from build123d import *

# Parameters (mm, degrees)
F0_W        = 59
F0_H        = 41
F1_DEPTH    = 22
F2_R        = 15
F3_DEPTH    = 76.2
F4_T        = 0.5
F4_T4_ANGLE = 180.000000001
F4_T6_ANGLE = 180.000000001


# Not quite as in the source:
# - a shell that OpenCascade refuses in one call is made with other operations: the cavity is built on its own and cut out


with BuildPart() as f1:
    # F0 (on Front) → F1 (new body)
    with BuildSketch(Plane.XZ):
        Rectangle(F0_W, F0_H)
    extrude(amount=-F1_DEPTH)

    # F2 (on Front) → F3 (join)
    with BuildSketch(Plane.XZ):
        with Locations((-14.5, 0)):
            Circle(F2_R)
    extrude(amount=-F3_DEPTH)

    # F4: shell of thickness 0.5, made by hand


with BuildPart() as f4_core1:
    # F4_t2: copy of F1
    add(f1.part)

    # the walls: a layer under each face that stays
    f4_faces = [f4_core1.faces().sort_by_distance(p)[0] for p in [
        (29.5, 11, 0),
        (0, 22, -13.6666666667),
        (-29.5, 49.1, 0),
        (-14.5, 76.2, 0),
        (-29.5, 11, 0),
        (0, 11, 20.5),
        (0, 11, -20.5),
    ]]
    thicken(f4_faces, amount=-F4_T, mode=Mode.SUBTRACT)

    # F4_s3 → F4_t4 (revolve, cut)
    with BuildSketch(Plane.XY):
        Polygon((-29.505, 22.005), (-29.5, 21.5), (-29, 21.5), (-29, 22), align=None)
    revolve(axis=Axis((-14.5, 22, 0), (0, -1, 0)), revolution_arc=F4_T4_ANGLE, mode=Mode.SUBTRACT)

    # F4_s5 → F4_t6 (revolve, cut)
    with BuildSketch(Plane.XY):
        Polygon((0.505, 22.005), (0.5, 21.5), (0, 21.5), (0, 22), align=None)
    revolve(axis=Axis((-14.5, 22, 0), (0, -1, 0)), revolution_arc=F4_T6_ANGLE, mode=Mode.SUBTRACT)


with BuildPart() as f1_1:
    add(f1.part)

    # what is left inside the walls is the cavity
    f4_cavity = [f4_core1.part.solids().sort_by_distance(p)[0] for p in [
        (-28.995, 57.8, 0),
    ]]
    add(f4_cavity, mode=Mode.SUBTRACT)


solid = f1_1.part
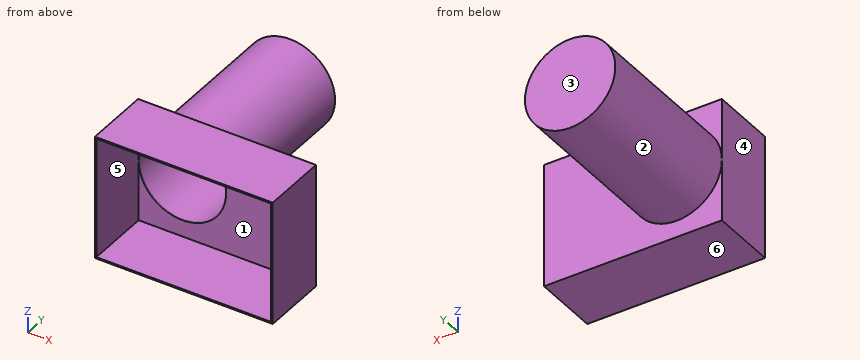
Geometry: final body of the model. Coordinates: model frame, mm. Face numbers are marked on the shaded views. A direction names the side the tool comes from. Give positions to 0.01 mm unless a question says otherwise; leave off trailing zeros. Loops run counter-clockwise (first coordinate to the right, second up) from the corner with the lowest first, then second, coordinate; pieces in that order, holes last. Notation, with made-up numbers: (17, -10.5) - (73, -10.5) arc R17 ccw to (73, 18.5) - close; hole circle Ø10 at (49.5, 28.25). An arc over 180 degrees is marked (long way). Answer as CSV lines item,"result". Start each with the question number.
1. Section D-D, the plane x = 10.5. Return loops of the section in (y, z), plus the area to 3 significant figures.
2. Reachability of the marked faces 1, 2 and 3 from +Z, -Z, +X, -X, +Y, -Y: full face, straight path, thin tool, end or side. Return the list, or none.
3. Section C-C, the plane z = -4.5. Return loops of the section in (x, y).
4. Draft query along Z for the marked faces 4, 5 and 6. Return one class per face: released by +Z, released by -Z, zero draft, split by the parting line, or undercut.
5. Section A-A, the plane y = 9. Return loops of the section in (x, z).
6. Section B-B, the plane x = -14.5. Return loops of the section in (y, z), plus the area to 3 significant figures.
7. Ray query, L1, parallel to X at y = 58, z = 0; L2, parallel to Z at x = -14.5, y = 56; L3, parallel to X at y = 6.5, z = 11.5. Return the intervals inside material, ascending.
8. Pin query (flat end, axial travel): P1, Ø6, axis at y = 48, z = -11, coming from the +X side; P2, Ø4, axis at x = 11.5, z = -3, coming from the -Y side; P3, Ø2, axis at x = -5, y = 39.5, coming from the -Z side. Return the tip coordinate at first contact, or that it passes through.
Answers:
1,outline,"(0, -20.5) - (22, -20.5) - (22, 20.5) - (0, 20.5) - (0, 20) - (21.5, 20) - (21.5, -20) - (0, -20) - close"
1,area,"42.0 mm2"
2,face 1,"-Y"
2,face 2,"+Y"
2,face 3,"+Z, -Z, +X, -X, +Y"
3,outline,"(-29.5, 0) - (-29, 0) - (-29, 21.5) - (-28.28, 21.5) - (-28.28, 75.7) - (-0.72, 75.7) - (-0.72, 21.5) - (29, 21.5) - (29, 0) - (29.5, 0) - (29.5, 22) - (-0.19, 22) - (-0.19, 76.2) - (-28.81, 76.2) - (-28.81, 22) - (-29.5, 22) - close"
4,face 4,"zero draft"
4,face 5,"undercut"
4,face 6,"released by -Z"
5,outline,"(-29.5, -20.5) - (29.5, -20.5) - (29.5, 20.5) - (-29.5, 20.5) - close; hole (-29, -20) - (29, -20) - (29, 20) - (-29, 20) - close"
6,outline,"(0, -20.5) - (22, -20.5) - (22, -15) - (76.2, -15) - (76.2, 15) - (22, 15) - (22, 20.5) - (0, 20.5) - (0, 20) - (21.5, 20) - (21.5, 14.5) - (75.7, 14.5) - (75.7, -14.5) - (21.5, -14.5) - (21.5, -20) - (0, -20) - close"
6,area,"96.2 mm2"
7,L1,"x = -29.5 to -29, 0 to 0.5"
7,L2,"z = -15 to -14.5, 14.5 to 15"
7,L3,"x = -29.5 to -29, 29 to 29.5"
8,P1,"stops at x = -1.81"
8,P2,"stops at y = 21.5"
8,P3,"stops at z = -12.36"
